Input: dimensioned drawing with shaded views. Units: mm. Origin: part minimum x, y, z. A direction names the side the tool comes from. Coordinates: 2 decimals unless noted, no trailing zeros. Order: outer loops, then holes, each group sorted by start corner. A loop starts at its lowest first (then second) coordinate and runs counter-clockwise, first axis right, second up.
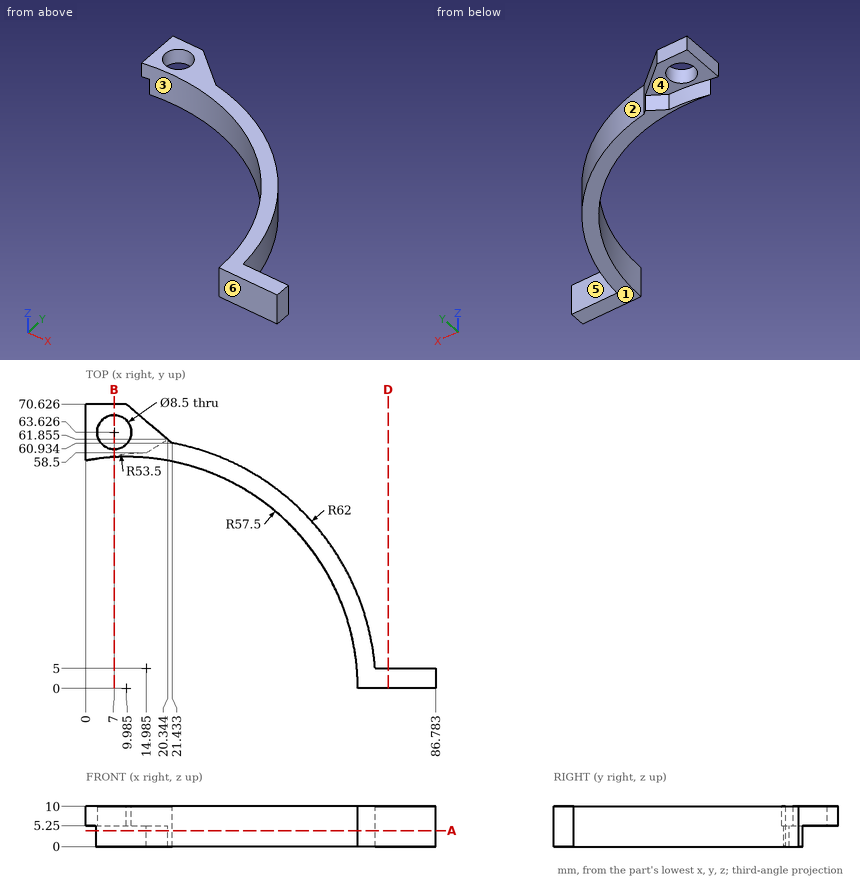
1. Pin query (flat end, axial travel): P1, Ø5, axis at x = 82.5, z = 6.5, coming from the +Y side; P2, Ø5, axis at y = 33.5, z = 4, coming from the +X side; P3, Ø7, axis at x = 6, y = 66, coming from the -Z side. Return the tip coordinate at first contact, or that it passes through.
Findings:
P1: stops at y = 5
P2: stops at x = 63.68
P3: stops at z = 5.25
2. Draft query along X for the marked faces 1, 2 and 3. Return one class per face: released by +X, released by -X, zero draft, split by the parting line, or undercut.
Findings:
face 1: zero draft
face 2: released by +X
face 3: undercut
3. Section query A-A on z = 4. Return loops of the section in (x, y) (1 decimal).
Findings:
outline: (2.4, 57) arc R57.5 cw to (67.5, 0) - (86.8, 0) - (86.8, 5) - (71.8, 5) arc R62 ccw to (21.4, 60.9) - (20.3, 61.9) - (15, 58.5) arc R53.5 ccw to start
4. Section query D-D on x = 75. Return loops of the section in (y, z), plus the area to 3 significant figures.
Findings:
outline: (0, 0) - (5, 0) - (5, 10) - (0, 10) - close
area: 50.0 mm2
5. Section query B-B on x = 7. Return loops of the section in (y, z).
Findings:
outline: (57.42, 0) - (57.9, 0) - (57.9, 5.25) - (59.38, 5.25) - (59.38, 10) - (57.42, 10) - close; (67.88, 5.25) - (70.63, 5.25) - (70.63, 10) - (67.88, 10) - close
6. Ray query, line 1 (Y direction, x = 81, z = 7.5); line 2 (Y direction, x = 7, z = 7.75); line 3 (Y direction, x = 9, z = 5.5) (1 decimal). Return the intervals inside material, ascending.
Findings:
line 1: y = 0 to 5
line 2: y = 57.42 to 59.38, 67.88 to 70.63
line 3: y = 57.5 to 59.9, 67.4 to 70.6
7. Access query for the marked faces 4, 5 and 6. Directions: +Z, -Z, +X, -X, +Y, -Y. A direction counts if a zero-diameter tool reaches every point of the face in a straight line with its end or side. Return the directions, or none.
Findings:
face 4: -Z, -X, +Y
face 5: +Z, -Z, +X, +Y
face 6: +Z, -Z, +X, -X, -Y
